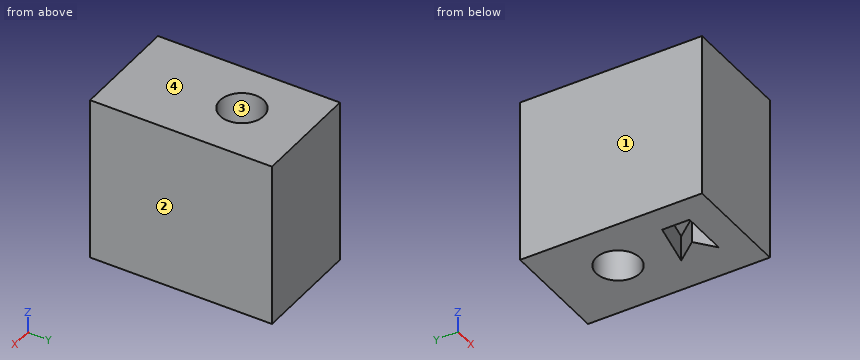
from build123d import *

# Parameters (mm, degrees)
F0_W      = 30
F0_H      = 50
F1_DEPTH  = 25.4
F1_FACE_W = 30
F1_FACE_H = 50
F2_DEPTH  = 20
F4_D      = 12
F6_DEPTH  = 7


with BuildPart() as f1:
    # F0 (on Top) → F1 (new body)
    with BuildSketch(Plane.XY):
        with Locations((-22.883214, -2.406316)):
            Rectangle(F0_W, F0_H)
    extrude(amount=F1_DEPTH)

    # F1_face (on face) → F2 (join)
    with BuildSketch(Plane(origin=(-22.883214, -2.406316, 25.4), x_dir=(1, 0, 0), z_dir=(0, 0, 1))):
        Rectangle(F1_FACE_W, F1_FACE_H)
    extrude(amount=F2_DEPTH)

    # F4 (through all)
    with Locations(Plane.XY.offset(45.4)):
        with Locations((-23.912763, 4.361447)):
            Hole(F4_D / 2)

    # F5 (on Top) → F6 (cut)
    with BuildSketch(Plane.XY):
        Polygon((-17.755329, -9.173958), (-30.53013, -11.881185), (-30.53013, -19.400921), (-22.709606, -19.400921), (-17.596183, -19.400921), (-22.709606, -15.189869), align=None)
    extrude(amount=F6_DEPTH, mode=Mode.SUBTRACT)


solid = f1.part
Can you work these out from the model? Positions are in its coordinate system, mm. Face numbers are marked on the shaded views. Give positions to 0.01 mm unless a question says otherwise; leave off trailing zeros. Loops run counter-clockwise (first coordinate to the right, second up) from the corner with the lowest first, then second, coordinate; pieces in that order, holes last. Notation, with made-up numbers: M 17.5,74 L 37.5,74 A27 cw 37.5,97 Z; hole C 7,19.25 d9. An arc over 180 degrees is marked long. One line per item, written item: value. Start each with the question number.
1) If I drill on line 1 (Y direction, x = -23.5, z = 10.5); line 2 (X direction, y = 4, z = 8); line 3 (X direction, y = 6, z = 14), over which ranges is the centre line in solid material (lowest first)? Write a range as [from, to].
2) I'm going to push a flat-ended pin straight in: pin 1 (5 mm diameter, centred on x = -27, y = -16.5, fed in from -Z). Where does the tip first touch, or does it pass through?
3) Thinking about a two-plate mould opening in X: for the marked faces 1, 2, 3 and 4, which applies, +X half, -X half, draft (parallel to the pull), parting line (faces both ways), or undercut?
4) If we section it at B-B, the plane y = 6.5: Write out the boundary of the cut face in (x, z), and give its area (3 significant figures).
5) If we section it at C-C, the plane z = 5: Write out the boundary of the cut face in (x, y).
6) If we section it at D-D, the plane z = 12: Write out the boundary of the cut face in (x, y), and give its area (3 significant figures).
7) If we section it at A-A, the plane x = -27.25: Write out the boundary of the cut face in (y, z).
Completed:
1. line 1: y = [-27.41, -1.62], [10.35, 22.59]
1. line 2: x = [-37.88, -29.9], [-17.92, -7.88]
1. line 3: x = [-37.88, -29.68], [-18.14, -7.88]
2. pin 1: stops at z = 7
3. face 1: -X half
3. face 2: +X half
3. face 3: undercut
3. face 4: draft
4. outline: M -37.88,0 L -29.52,0 L -29.52,45.4 L -37.88,45.4 Z; M -18.31,0 L -7.88,0 L -7.88,45.4 L -18.31,45.4 Z
4. area: 853 mm^2
5. outline: M -37.88,-27.41 L -7.88,-27.41 L -7.88,22.59 L -37.88,22.59 Z; hole M -30.53,-19.4 L -17.6,-19.4 L -22.71,-15.19 L -17.76,-9.17 L -30.53,-11.88 Z; hole C -23.91,4.36 d12
6. outline: M -37.88,-27.41 L -7.88,-27.41 L -7.88,22.59 L -37.88,22.59 Z; hole C -23.91,4.36 d12
6. area: 1,390 mm^2
7. outline: M -27.41,0 L -19.4,0 L -19.4,7 L -11.19,7 L -11.19,0 L -0.62,0 L -0.62,45.4 L -27.41,45.4 Z; M 9.35,0 L 22.59,0 L 22.59,45.4 L 9.35,45.4 Z
